Geometry: see drawing. Coordinates: mm, zero at the bounding-box minimum. A direction names the side the tool comes from. Round coordinates to 2 decimals unless told otherwise and drop trailing zeros. Order: outer loops, then holes, each group sorted by start corner. A loop starts at its lowest first (then second) coordinate and runs counter-clockwise, first axis right, second up. Notation, with made-up numbers: (-32.75, 85) - (20.25, 85) arc R19 cw to (20.25, 115) - close; hole circle Ø7 at (-2.5, 72.5). An arc over 180 degrees is marked (long way). Put each result on its own line as item: value. Start each with the question number.
1) Contact query for flat-ended pins moving along their axis: P1, Ø2, axis at x = 2, y = 7.5, coming from the +Z side; P2, Ø4, axis at x = 7, z = 10, coming from the -Y side; P3, Ø4, axis at x = 3, z = 4, coming from the +Y side. Output: stop coordinate, or through.
2) Line query: probe 1 along Z at (x, y) = (8.5, 6); probe 2 along Z at (x, y) = (3.5, 4.5) (1 decimal); probe 3 along Z at (x, y) = (9.5, 5.5). Output: solid intervals per line, ascending. Write a range as [from, to].
3) Section B-B on z = 2. Output: boundary loops of the cut face in (x, y).
4) Section A-A on z = 6. Output: boundary loops of the cut face in (x, y).
5) Access query for the marked faces 4, 5 and 6. Directions: +Z, -Z, +X, -X, +Y, -Y. A direction counts if a zero-diameter tool reaches every point of the face in a straight line with its end or side. Return the directions, or none.
6) Mould query, pull axis Z, two halves, no side actions, for the marked faces 1, 2 and 3. Classes: +Z half, -Z half, draft (parallel to the pull), parting line (faces both ways), or undercut.
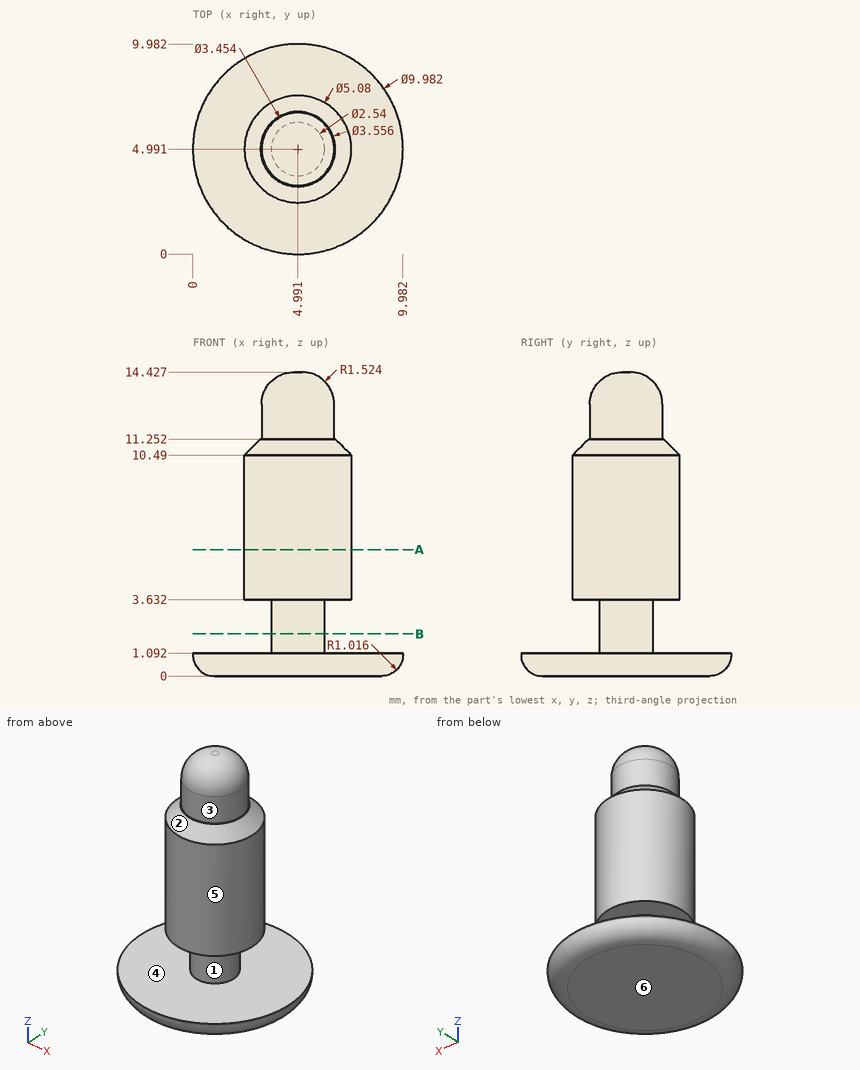
Answer sheet:
1. P1: z = 1.09
1. P2: y = 2.45
1. P3: y = 7.53
2. probe 1: [0, 1.09]
2. probe 2: [0, 1.1], [3.6, 13.6]
2. probe 3: [0.17, 1.09]
3. outline: circle Ø2.54 at (4.99, 4.99)
4. outline: circle Ø5.08 at (4.99, 4.99)
5. face 4: none
5. face 5: +Z
5. face 6: -Z, +X, -X, +Y, -Y
6. face 1: undercut
6. face 2: +Z half
6. face 3: draft
